from build123d import *

# Parameters (mm, degrees)
F0_W     = 55.5625
F0_H     = 68.2625
F0_H_2   = 96.8375
F1_DEPTH = 15
F3_DEPTH = 10
F4_W     = 20
F4_H     = 5
F5_DEPTH = 25
F6_W     = 20
F6_H     = 8
F7_DEPTH = 15


with BuildPart() as f1:
    # F0 (on Top) → F1 (new body)
    with BuildSketch(Plane.XY):
        with Locations((0, -48.41875)):
            Rectangle(F0_W, F0_H)
        Polygon((27.78125, -14.2875), (27.78125, -82.55), (40.48125, -82.55), align=None)
        Polygon((-40.48125, -82.55), (-27.78125, -82.55), (-27.78125, -14.2875), align=None)
        with Locations((0, 34.13125)):
            Rectangle(F0_W, F0_H_2)
    extrude(amount=F1_DEPTH)

    # F2 (on face) → F3 (cut)
    with BuildSketch(Plane(origin=(0, 0, 0), x_dir=(1, 0, 0), z_dir=(0, 0, -1))):
        Polygon((34.4403, 79.25), (-35.392648, 79.25), (-24.48125, 14.2875), (-24.48125, -79.25), (24.482846, -79.25), (24.482846, 14.390121), align=None)
    extrude(amount=-F3_DEPTH, mode=Mode.SUBTRACT)

    # F4 (on face) → F5 (cut)
    with BuildSketch(Plane.XZ.offset(82.55)):
        with Locations((0, 7.5)):
            Rectangle(F4_W, F4_H)
    extrude(amount=-F5_DEPTH, mode=Mode.SUBTRACT)

    # F6 (on face) → F7 (join)
    with BuildSketch(Plane(origin=(0, 82.55, 0), x_dir=(-1, 0, 0), z_dir=(0, 1, 0))):
        with Locations((0, 7.5)):
            Rectangle(F6_W, F6_H)
    extrude(amount=F7_DEPTH)


solid = f1.part
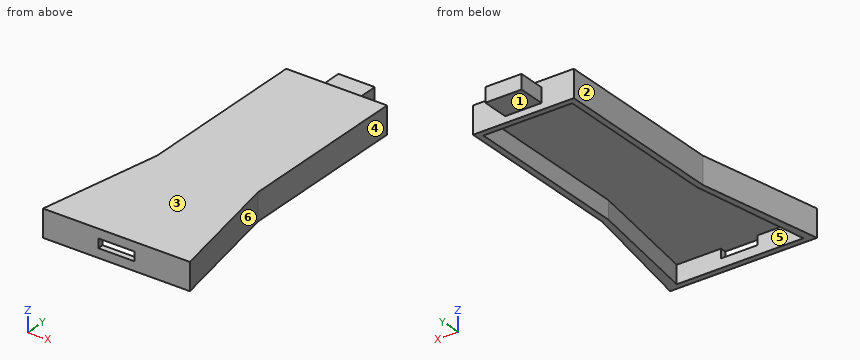
Input: part model. Units: mm. Frame: model coordinates. Face numbers are marked on the shaded views. A direction names the side the tool comes from. Give positions to 0.01 mm unless a question says otherwise; leave off trailing zeros. Loops run counter-clockwise (first coordinate to the right, second up) from the corner with the lowest first, then second, coordinate; pieces in that order, holes last. Notation, with made-up numbers: (65.25, -23) -> (122.25, -23) arc R23 cw to (122.25, 7) -> close; hole circle Ø11 at (-13.75, 13.25). An arc over 180 degrees is marked (long way). Answer as a JSON object with one key per item and string values. Group by question number.
Item 1: Pull-direction query (Y, two-part tool) for the marked faces 4, 5 and 6; classes: released by +Y, released by -Y, zero draft, split by the parting line, or undercut.
Item 2: Reachability of the marked faces 1, 2 and 3 from +Z, -Z, +X, -X, +Y, -Y: full face, straight path, thin tool, end or side. Return the list, or none.
Item 3: Cut plane A-A, the plane x = 8. Return the cut outline in (y, z).
Item 4: Cut plane C-C, the plane x = 29.5. Return the cut outline in (y, z), and give its area (3 significant figures).
Item 5: Line query: probe 1 along X at (y, z) = (44, 2.25); probe 2 along Y at (x, z) = (17, 3.75); probe 3 along Y at (x, z) = (4.5, 9.5). Output: solid intervals per line, ascending.
Item 6: Pin query (flat end, axial travel): P1, Ø6, axis at x = -2, y = -53.5, coming from the -Z side; P2, Ø5, axis at y = -59.5, z = 5, coming from the -X side; P3, Ø7.5, axis at x = 3, y = 92, coming from the +Z side. Return the tip coordinate at first contact, or that it passes through.
Item 7: Cut plane B-B, the plane y = -7. Return the cut outline in (x, z), and give its area (3 significant figures).
Checks:
{
 "1": {"face 4": "zero draft", "face 5": "undercut", "face 6": "released by +Y"},
 "2": {"face 1": "-Z, +X, -X, +Y", "face 2": "+Z, -Z, -X, +Y", "face 3": "+Z, +X, -X, +Y, -Y"},
 "3": {"outline": "(-82.55, 0) -> (-79.25, 0) -> (-79.25, 5) -> (-82.55, 5) -> close; (-82.55, 10) -> (79.25, 10) -> (79.25, 0) -> (82.55, 0) -> (82.55, 3.5) -> (97.55, 3.5) -> (97.55, 11.5) -> (82.55, 11.5) -> (82.55, 15) -> (-82.55, 15) -> close"},
 "4": {"outline": "(-82.55, 0) -> (-79.25, 0) -> (-79.25, 10) -> (-47.07, 10) -> (-47.07, 0) -> (-23.53, 0) -> (-23.53, 15) -> (-82.55, 15) -> close", "area": "564 mm²"},
 "5": {"probe 1": "x = -27.78 to -24.48, 24.48 to 27.78", "probe 2": "y = -82.55 to -79.25, 79.25 to 82.55", "probe 3": "y = 79.25 to 97.55"},
 "6": {"P1": "stops at z = 10", "P2": "stops at x = -36.66", "P3": "stops at z = 11.5"},
 "7": {"outline": "(-27.78, 0) -> (-24.48, 0) -> (-24.48, 10) -> (24.48, 10) -> (24.48, 0) -> (27.78, 0) -> (27.78, 15) -> (-27.78, 15) -> close", "area": "344 mm²"}
}
